from build123d import *

# Parameters (mm, degrees)
SKETCH1_R           = 12.192
SKETCH1_R_2         = 9.017
CORE_EXTRUDE_DEPTH  = 79.375
GROOVE_CUT_DEPTH    = 19.05
BUMPY_START         = -3.175
SKETCH3_R           = 9.017
BUMPY_EXTRUDE_DEPTH = 3.175
SKETCH7_R           = 1.11125
CUT_EXTRUDE3_DEPTH  = 79.126370247


with BuildPart() as part:
    # Sketch1 → Core Extrude (new body)
    with BuildSketch(Plane.XY):
        with Locations(Location((0, 0, 0), (0, 0, 180))):
            Circle(SKETCH1_R)
        with Locations(Location((0, 0, 0), (0, 0, 180))):
            Circle(SKETCH1_R_2, mode=Mode.SUBTRACT)
    extrude(amount=CORE_EXTRUDE_DEPTH)

    # Sketch2 → Groove Cut (cut)
    with BuildSketch(Plane(origin=(0, 0, 0), x_dir=(-1, 0, 0), z_dir=(0, 0, -1))):
        with BuildLine():
            ThreePointArc((-8.439529845, -3.175), (-9.017, 0), (-8.439529845, 3.175))
            ThreePointArc((-8.439529845, 3.175), (-10.922, 0), (-8.439529845, -3.175))
        make_face()
        with BuildLine():
            ThreePointArc((-3.175, 8.439529845), (0, 9.017), (3.175, 8.439529845))
            ThreePointArc((3.175, 8.439529845), (0, 10.922), (-3.175, 8.439529845))
        make_face()
        with BuildLine():
            ThreePointArc((8.439529845, -3.175), (10.922, 0), (8.439529845, 3.175))
            ThreePointArc((8.439529845, 3.175), (8.871457874, 1.613543986), (9.017, 0))
            ThreePointArc((9.017, 0), (8.871457874, -1.613543986), (8.439529845, -3.175))
        make_face()
        with BuildLine():
            ThreePointArc((-3.175, -8.439529845), (0, -10.922), (3.175, -8.439529845))
            ThreePointArc((3.175, -8.439529845), (0, -9.017), (-3.175, -8.439529845))
        make_face()
    extrude(amount=-GROOVE_CUT_DEPTH, mode=Mode.SUBTRACT)

    # Sketch3 → Bumpy Extrude (add)
    with BuildSketch(Plane.XY.offset(79.375).offset(BUMPY_START)):
        with Locations(Location((0, 0, 0), (0, 0, 159.383409617))):
            Circle(SKETCH3_R)
    extrude(amount=BUMPY_EXTRUDE_DEPTH)

    # Sketch5 → Revolve1 (revolve)
    with BuildSketch(Plane(origin=(0, 0, 0), x_dir=(0, 0, -1), z_dir=(1, 0, 0))):
        with BuildLine():
            Line((-88.9, 0), (-79.375, 0))
            Line((-79.375, 0), (-79.375, 6.35))
            Line((-79.375, 6.35), (-82.55, 6.35))
            ThreePointArc((-82.55, 6.35), (-87.040128061, 4.490128061), (-88.9, 0))
        make_face()
    revolve(axis=Axis((0, 0, 79.375), (0, 0, 1)))

    # Sketch7 → Cut-Extrude3 (cut, through all)
    with BuildSketch(Plane(origin=(0, 0, 76.2), x_dir=(-1, 0, 0), z_dir=(0, 0, -1))):
        Circle(SKETCH7_R)
    extrude(amount=-CUT_EXTRUDE3_DEPTH, mode=Mode.SUBTRACT)


solid = part.part
Work out the finished part from the listing and answer in its coordinate system (mm). A direction names the side the tool comes from. Give positions to 0.01 mm unless a question says otherwise; leave off trailing zeros. Order: outer loops, then holes, each group sorted by start corner. A loop starts at its lowest first (then second) coordinate and runs counter-clockwise, first axis right, second up. Notation, with made-up numbers: (-3, 47.25) -> (3, 47.25) arc R18 ccw to (3, 66.25) -> close; hole circle Ø3 at (24, -39.75). An arc over 180 degrees is marked (long way). Answer as a JSON object with one key per item and string values. Group by question number.
1. Flat-ended cylindrical pins translate along their axes: pin 1 Ø12 at (y, z) = (9.5, 26) entering from -X; pin 2 Ø14.5 at (x, y) = (0, 0) entering from -Z; pin 3 Ø5 at (x, z) = (6.5, 16) entering from -Y. Find the tip coordinate at first contact, or state that the pin passes through.
2. A tool of negligible diameter and unlimited length cuts with its end or side. For faces 1 (the flat face through (1, 2, 76.2)), 2 (the flat face through (-8.1, 4.5, 0)), from which of +Z, -Z, +X, -X, +Y, -Y can it reach the whole face along a straight path? Write none if from no direction.
3. Section A-A on y = 0 is taken. Determine the outline of the cut face in (x, z) (3 decimals), plus the area to 3 significant figures.
4. Section C-C on z = 36 is taken. Determine the outline of the cut face in (x, y), plus the area to 3 significant figures.
5. Consider line 1 along Y through (x, z) = (0, 29); line 2 along Y through (x, z) = (0, 82.5); line 3 along Z through (x, y) = (-9.5, -5.75) (3 decimals). Determine where each line is inside the solid, lowest interval first. Write a range as [from, to].
6. Section D-D on y = 4.25 is taken. Determine the outline of the cut face in (x, z) (3 decimals).
7. The mould has two halves that part along X. Classify faces 3 (the cylindrical face through (0.06, -10.92, 9.39)), 4 (the flat face through (-5, 5, 79.375)), 5 (the cylindrical face through (6.2, -1.38, 80.98)): released by +X, released by -X, zero draft, split by the parting line, or undercut.
Result sheet:
{
 "1": {"pin 1": "stops at x = -11.68", "pin 2": "stops at z = 76.2", "pin 3": "stops at y = -11.52"},
 "2": {"face 1": "-Z", "face 2": "-Z, +X, -X, +Y, -Y"},
 "3": {"outline": "(-12.192, 0) -> (-10.922, 0) -> (-10.922, 19.05) -> (-9.017, 19.05) -> (-9.017, 76.2) -> (-1.111, 76.2) -> (-1.111, 88.802) arc R6.35 ccw to (-6.35, 82.55) -> (-6.35, 79.375) -> (-12.192, 79.375) -> close; (1.111, 76.2) -> (9.017, 76.2) -> (9.017, 19.05) -> (10.922, 19.05) -> (10.922, 0) -> (12.192, 0) -> (12.192, 79.375) -> (6.35, 79.375) -> (6.35, 82.55) arc R6.35 ccw to (1.111, 88.802) -> close", "area": "564 mm^2"},
 "4": {"outline": "circle Ø24.38 at (0, 0); hole circle Ø18.03 at (0, 0)", "area": "212 mm^2"},
 "5": {"line 1": "y = [-12.19, -9.02], [9.02, 12.19]", "line 2": "y = [-6.35, -1.11], [1.11, 6.35]", "line 3": "z = [0, 79.375]"},
 "6": {"outline": "(-11.427, 0) -> (-7.953, 0) -> (-7.953, 76.2) -> (7.953, 76.2) -> (7.953, 0) -> (11.427, 0) -> (11.427, 79.375) -> (4.718, 79.375) -> (4.718, 82.55) arc R4.718 ccw to (-4.718, 82.55) -> (-4.718, 79.375) -> (-11.427, 79.375) -> close"},
 "7": {"face 3": "undercut", "face 4": "zero draft", "face 5": "split by the parting line"}
}
